For this review, take the finished solid that the model builds, in its own axes (mm). Face numbers are marked on the shaded views. A direction names the side the tool comes from. Give positions to 0.01 mm unless a question says otherwise; leave off trailing zeros. Loops run counter-clockwise (first coordinate to the right, second up) from the corner with the lowest first, then second, coordinate; pieces in that order, holes last. Notation, with made-up numbers: (-13.75, -12.75) -> (31.25, -12.75) arc R26 cw to (31.25, 7.25) -> close; hole circle Ø2 at (-12.5, -3). An arc over 180 degrees is marked (long way). Write each question's results on one line, items separated by ' | '. Start each with the question number.
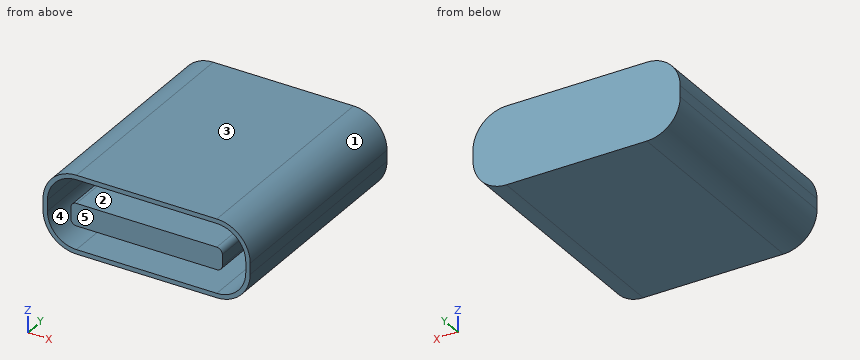
Autodesk Inventor part; units mm, degrees
ref_plane "YZ Plane" through (0, 0, 0) normal (1, 0, 0) x (0, 1, 0)
ref_plane "XZ Plane" through (0, 0, 0) normal (0, 1, 0) x (-1, 0, 0)
ref_plane "XY Plane" through (0, 0, 0) normal (0, 0, 1) x (1, 0, 0)
ref_plane "Work Plane1" through (0, 0, 0) normal (0, 0, 1) x (1, 0, 0)
sketch "Sketch1" plane through (0, 0, 0) normal (0, 0, 1) x (1, 0, 0)
  line L0 (6.3465, -41.9537) -> (15.6465, -41.9537)
  line L1 (15.6465, -41.9537) -> (15.6465, -51.9537)
  line L2 (15.6465, -51.9537) -> (6.3465, -51.9537)
  line L3 (6.3465, -51.9537) -> (6.3465, -41.9537)
  point P0 (0, 0)
  dimension "d0" = 9.3
  dimension "d2" = 10
extrude "Extrusion1" add sketch "Sketch1" along normal blind 3.5
fillet "Fillet1" radius 1.5 4 edges at (15.6465, -46.9537, 3.5) (6.3465, -46.9537, 3.5) (6.3465, -46.9537, 0) (15.6465, -46.9537, 0)
shell "Shell1" thickness 0.2 removed faces 1 at (9.9465, -51.9537, 2.3333)
sketch "Sketch2" plane through (7.8465, -42.1537, 3.3) normal (0, -1, 0) x (1, 0, 0)
  arc A0 (6.3, -3.1) -> (7.6, -1.8) centre (6.3, -1.8) ccw
  line L0 (7.6, -1.8) -> (7.6, -1.3)
  arc A1 (7.6, -1.3) -> (6.3, 0) centre (6.3, -1.3) ccw
  line L1 (6.3, 0) -> (0, 0)
  arc A2 (0, 0) -> (-1.3, -1.3) centre (0, -1.3) ccw
  line L2 (-1.3, -1.8) -> (-1.3, -1.3)
  arc A3 (-1.3, -1.8) -> (0, -3.1) centre (0, -1.8) ccw
  line L3 (0, -3.1) -> (6.3, -3.1)
  line L4 (0, -1.05) -> (6.3, -1.05)
  arc A4 (6.55, -1.3) -> (6.3, -1.05) centre (6.3, -1.3) ccw
  line L5 (6.55, -1.3) -> (6.55, -1.8)
  arc A5 (6.3, -2.05) -> (6.55, -1.8) centre (6.3, -1.8) ccw
  line L6 (6.3, -2.05) -> (0, -2.05)
  arc A6 (-0.25, -1.8) -> (0, -2.05) centre (0, -1.8) ccw
  line L7 (-0.25, -1.8) -> (-0.25, -1.3)
  arc A7 (0, -1.05) -> (-0.25, -1.3) centre (0, -1.3) ccw
  point P0 (-7.8465, -3.3)
  dimension "d7" = 1
extrude "Extrusion2" add sketch "Sketch2" along normal up to surface (9.8 mm away) contours L4 A4 L5 A5 L6 A6 L7 A7
properties part number "nanopc_t4_usb3c"
1. We need section A-A (y = -43.25). Write out the cut boundary in (x, z).
2. We need section B-B (z = 1.65). Write out the cut boundary in (x, y).
3. Draft analysis for pull direction Z (two halves, no side actions). For the marked faces 3, 4 and 5, state which applies: released by +Z, released by -Z, zero draft, split by the parting line, or undercut.
4. Wall thickness on L1, parallel to Z at x = 10.5, y = -43.25; L2, parallel to X at y = -46.5, z = 1.55; L3, parallel to X at y = -43, z = 0.6: over which ranges is each line inside the solid? List them lowest first.
5. We need section D-D (z = 1). Write out the cut boundary in (x, y), plus the area to 3 significant figures.
6. Machinability: for the marked faces 1 and 2, which of the approach directions +Z, -Z, +X, -X, +Y, -Y give a long, thin tool a straight path to every point of the face, cutting with its end or side? Answer none if there is none.
7. We need section C-C (x = 10.75). Write out the cut boundary in (y, z), plus the area to 3 significant figures.
Response:
1) outline: (6.35, 1.5) arc R1.5 ccw to (7.85, 0) -> (14.15, 0) arc R1.5 ccw to (15.65, 1.5) -> (15.65, 2) arc R1.5 ccw to (14.15, 3.5) -> (7.85, 3.5) arc R1.5 ccw to (6.35, 2) -> close; (7.6, 1.5) arc R0.25 ccw to (7.85, 1.25) -> (14.15, 1.25) arc R0.25 ccw to (14.4, 1.5) -> (14.4, 2) arc R0.25 ccw to (14.15, 2.25) -> (7.85, 2.25) arc R0.25 ccw to (7.6, 2) -> close; hole (6.55, 1.5) arc R1.3 ccw to (7.85, 0.2) -> (14.15, 0.2) arc R1.3 ccw to (15.45, 1.5) -> (15.45, 2) arc R1.3 ccw to (14.15, 3.3) -> (7.85, 3.3) arc R1.3 ccw to (6.55, 2) -> close
2) outline: (6.35, -51.95) -> (6.55, -51.95) -> (6.55, -42.15) -> (7.6, -42.15) -> (7.6, -51.95) -> (14.4, -51.95) -> (14.4, -42.15) -> (15.45, -42.15) -> (15.45, -51.95) -> (15.65, -51.95) -> (15.65, -41.95) -> (6.35, -41.95) -> close
3) face 3: released by +Z | face 4: undercut | face 5: zero draft
4) L1: z = 0 to 0.2, 1.25 to 2.25, 3.3 to 3.5 | L2: x = 6.35 to 6.55, 7.6 to 14.4, 15.45 to 15.65 | L3: x = 6.65 to 6.91, 15.08 to 15.35
5) outline: (6.43, -51.95) -> (6.65, -51.95) -> (6.65, -42.15) -> (15.35, -42.15) -> (15.35, -51.95) -> (15.56, -51.95) -> (15.56, -41.95) -> (6.43, -41.95) -> close | area: 6.02 mm2
6) face 1: +Z, +X, +Y, -Y | face 2: -Y
7) outline: (-51.95, 0) -> (-41.95, 0) -> (-41.95, 3.5) -> (-51.95, 3.5) -> (-51.95, 3.3) -> (-42.15, 3.3) -> (-42.15, 2.25) -> (-51.95, 2.25) -> (-51.95, 1.25) -> (-42.15, 1.25) -> (-42.15, 0.2) -> (-51.95, 0.2) -> close | area: 14.4 mm2
